Here's how the part is built. I have some questions about the finished solid (model axes, mm). A direction names the side the tool comes from. Coordinates: 2 decimals unless noted, no trailing zeros. Use a Markdown table: item, result.
```python
from build123d import *

# Parameters (mm, degrees)
SKETCH1_R           = 1.15
SKETCH1_R_2         = 1.1
BOSS_EXTRUDE1_DEPTH = 2.5
SKETCH2_R           = 2.1
CUT_EXTRUDE1_DEPTH  = 1.5
SKETCH3_W           = 95.504738846
SKETCH3_H           = 6
BOSS_EXTRUDE2_DEPTH = 1.5
FILLET1_R           = 0.5
FILLET2_R           = 0.5
SKETCH4_R           = 2.1
SKETCH4_W           = 96.504738846
SKETCH4_H           = 7
CUT_EXTRUDE2_DEPTH  = 0.6


with BuildPart() as part:
    # Sketch1 → Boss-Extrude1 (new body)
    with BuildSketch(Plane(origin=(0.142209029, 4.250598455, 0), x_dir=(0.999440809, -0.033437529, 0), z_dir=(-0.033437529, -0.999440809, 0))):
        Polygon((11.443429389, 116.200036636), (14.167398509, 118.020989552), (14.167398349, 121.688114552), (12.943429389, 122.700036636), (11.443429389, 123.000036636), (9.639575481, 122.500036636), (-10.832601571, 113.00003089), (-134.806739216, 113.00003089), (-134.806739216, 108.000029776), (-149.556569968, 108.000029776), (-149.556569968, 102.000029776), (-134.806740003, 102.000029776), (-134.806740003, 97.00003089), (-10.832601571, 97.00003089), (9.643430674, 87.500036636), (11.443430674, 87.000036636), (12.943429388, 87.300036636), (14.167399777, 89.020989552), (14.167399616, 92.688114552), (11.443430674, 93.800036636), (-10.832601571, 104.00003089), (-10.832601571, 106.00003089), align=None)
        with Locations((11.443429389, 119.700036636)):
            Circle(SKETCH1_R, mode=Mode.SUBTRACT)
        with Locations((11.443430674, 90.300036636)):
            Circle(SKETCH1_R, mode=Mode.SUBTRACT)
        with Locations((-145.556569968, 105.000029776)):
            Circle(SKETCH1_R, mode=Mode.SUBTRACT)
        with Locations((-120.056569968, 105.00003089)):
            Circle(SKETCH1_R_2, mode=Mode.SUBTRACT)
    extrude(amount=BOSS_EXTRUDE1_DEPTH)

    # Sketch2 → Cut-Extrude1 (cut)
    with BuildSketch(Plane(origin=(0.058615208, 1.751996431, 0), x_dir=(0.999440809, -0.033437529, 0), z_dir=(-0.033437529, -0.999440809, 0))):
        with Locations((-145.556569968, 105.000029776)):
            Circle(SKETCH2_R)
        with Locations((-120.056569968, 105.00003089)):
            Circle(SKETCH2_R)
        with Locations((11.443429389, 119.700036636)):
            Circle(SKETCH2_R)
        with Locations((11.443430674, 90.300036636)):
            Circle(SKETCH2_R)
    extrude(amount=-CUT_EXTRUDE1_DEPTH, mode=Mode.SUBTRACT)

    # Sketch3 → Boss-Extrude2 (add)
    with BuildSketch(Plane(origin=(0.058615208, 1.751996431, 0), x_dir=(0.999440809, -0.033437529, 0), z_dir=(-0.033437529, -0.999440809, 0))):
        with Locations((-66.082119318, 105.00003089)):
            Rectangle(SKETCH3_W, SKETCH3_H)
    extrude(amount=BOSS_EXTRUDE2_DEPTH)

    # Fillet1
    fillet1_edges = [part.edges().sort_by_distance(p)[0] for p in [
        (-113.712218368, 5.558340404, 105.00003089),
        (-65.986551616, 3.961619186, 102.00003089),
        (-18.260884865, 2.364897967, 105.00003089),
        (-65.986551616, 3.961619186, 108.00003089),
        (-113.762374661, 4.05917919, 105.00003089),
        (-66.036707909, 2.462457971, 102.00003089),
        (-18.311041158, 0.865736753, 105.00003089),
        (-66.036707909, 2.462457971, 108.00003089),
    ]]
    fillet(fillet1_edges, radius=FILLET1_R)

    # Fillet2
    fillet2_edges = [part.edges().sort_by_distance(p)[0] for p in [
        (-72.636741689, 6.685508279, 97.00003089),
        (-134.589148324, 8.758202679, 99.500030333),
        (-141.959939325, 9.00480161, 102.000029776),
        (-149.330730325, 9.25140054, 105.000029776),
        (-141.959938931, 9.004801596, 108.000029776),
        (-134.589147538, 8.758202653, 110.500030333),
        (-72.636741296, 6.685508266, 113.00003089),
        (-72.720335117, 4.186906242, 113.00003089),
        (-134.672741359, 6.259600629, 110.500030333),
        (-142.043532753, 6.506199573, 108.000029776),
        (-149.414324146, 6.752798517, 105.000029776),
        (-142.043533146, 6.506199586, 102.000029776),
        (-134.672742146, 6.259600655, 99.500030333),
        (-72.72033551, 4.186906256, 97.00003089),
    ]]
    fillet(fillet2_edges, radius=FILLET2_R)

    # Sketch4 → Cut-Extrude2 (cut)
    with BuildSketch(Plane(origin=(0.058615208, 1.751996431, 0), x_dir=(0.999440809, -0.033437529, 0), z_dir=(-0.033437529, -0.999440809, 0))):
        Polygon((11.443429389, 116.200036636), (14.167398509, 118.020989552), (14.167398349, 121.688114552), (12.943429389, 122.700036636), (11.443429389, 123.000036636), (9.639575481, 122.500036636), (-10.832601571, 113.00003089), (-11.910083922, 112.50003089), (-134.306739216, 112.50003089), (-134.306739216, 107.500029776), (-149.056569968, 107.500029776), (-149.056569968, 102.500029776), (-134.306740003, 102.500029776), (-134.306740003, 97.50003089), (-11.91028813, 97.50003089), (-10.832601571, 97.00003089), (9.643430674, 87.500036636), (11.443430674, 87.000036636), (12.943429388, 87.300036636), (14.167399777, 89.020989552), (14.167399616, 92.688114552), (11.443430674, 93.800036636), (-10.832601571, 104.00003089), (-10.832601571, 106.00003089), align=None)
        with Locations((11.443430674, 90.300036636)):
            Circle(SKETCH4_R, mode=Mode.SUBTRACT)
        with Locations((-145.556569968, 105.000029776)):
            Circle(SKETCH4_R, mode=Mode.SUBTRACT)
        with Locations((-120.056569968, 105.00003089)):
            Circle(SKETCH4_R, mode=Mode.SUBTRACT)
        with Locations((-66.082119318, 105.00003089)):
            Rectangle(SKETCH4_W, SKETCH4_H, mode=Mode.SUBTRACT)
        with Locations((11.443429389, 119.700036636)):
            Circle(SKETCH4_R, mode=Mode.SUBTRACT)
    extrude(amount=-CUT_EXTRUDE2_DEPTH, mode=Mode.SUBTRACT)


solid = part.part
```
1. Will these pins go through, and if not, where does the flat tip stop? pin 1 Ø1.1 at (x, y) = (-79.5, 5) entering from +Z; pin 2 Ø6 at (x, z) = (-66.5, 108.5) entering from -Y; pin 3 Ø0.9 at (x, y) = (-139.5, 6.5) entering from -Z.
Answers follow:
| item | result |
|---|---|
| pin 1 | stops at z = 113 |
| pin 2 | stops at y = 2.38 |
| pin 3 | stops at z = 102 |
2. We'd pull the mould along X, two halves only. Please class faces 1 (the face through (-74, 5, 97)), 2 (the face through (11.08, 2.43, 117.65)): +X half, -X half, draft (parallel to the pull), parting line (faces both ways), or undercut.
Answers follow:
| item | result |
|---|---|
| face 1 | draft |
| face 2 | undercut |
3. I need wall thicknesses on probe 1 along Z at (x, y) = (-23, 4); probe 2 along Z at (x, y) = (-26.5, 1.5); probe 3 along Y at (x, z) = (-89, 109.5). Which ranges of each line are inside material? Lowest first, please.
Answers follow:
| item | result |
|---|---|
| probe 1 | z = 97 to 113 |
| probe 2 | z = 102.02 to 107.98 |
| probe 3 | y = 5.33 to 7.23 |
4. Which directions (+Z, -Z, +X, -X, +Y, -Y) give clear straight access to the entire face, cutting with the end or side of a thin tool? Please do faces 3 (the face through (-65.316, 3.797, 101.85)), 4 (the face through (-66.7, 4.3, 101.5)), 5 (the face through (-72, 5, 113)).
Answers follow:
| item | result |
|---|---|
| face 3 | -Z, -X, -Y |
| face 4 | -X, -Y |
| face 5 | +Z, -X, +Y, -Y |
